```python
from build123d import *

# Parameters (mm, degrees)
BOSS_EXTRUDE1_DEPTH = 300
BOSS_EXTRUDE2_DEPTH = 10
SKETCH3_R           = 5
CUT_EXTRUDE1_DEPTH  = 624.643527987


with BuildPart() as part:
    # Sketch1 → Boss-Extrude1 (new, symmetric)
    with BuildSketch(Plane(origin=(0, 0, 0), x_dir=(0, 0, -1), z_dir=(1, 0, 0))):
        with BuildLine():
            Line((-20, 25), (20, 25))
            ThreePointArc((20, 25), (23.535533906, 23.535533906), (25, 20))
            Line((25, 20), (25, -20))
            ThreePointArc((25, -20), (23.535533906, -23.535533906), (20, -25))
            Line((20, -25), (-20, -25))
            ThreePointArc((-20, -25), (-23.535533906, -23.535533906), (-25, -20))
            Line((-25, -20), (-25, 20))
            ThreePointArc((-25, 20), (-23.535533906, 23.535533906), (-20, 25))
        make_face()
        with BuildLine():
            Line((-20, 23), (20, 23))
            ThreePointArc((20, 23), (22.121320344, 22.121320344), (23, 20))
            Line((23, 20), (23, -20))
            ThreePointArc((23, -20), (22.121320344, -22.121320344), (20, -23))
            Line((20, -23), (-20, -23))
            ThreePointArc((-20, -23), (-22.121320344, -22.121320344), (-23, -20))
            Line((-23, -20), (-23, 20))
            ThreePointArc((-23, 20), (-22.121320344, 22.121320344), (-20, 23))
        make_face(mode=Mode.SUBTRACT)
    extrude(amount=BOSS_EXTRUDE1_DEPTH, both=True)

    # Sketch2 → Boss-Extrude2 (add)
    with BuildSketch(Plane(origin=(300, 0, 0), x_dir=(0, 0, -1), z_dir=(1, 0, 0))):
        with BuildLine():
            Line((-57.5, 25), (57.5, 25))
            ThreePointArc((57.5, 25), (61.035533906, 23.535533906), (62.5, 20))
            Line((62.5, 20), (62.5, -20))
            ThreePointArc((62.5, -20), (61.035533906, -23.535533906), (57.5, -25))
            Line((57.5, -25), (-57.5, -25))
            ThreePointArc((-57.5, -25), (-61.035533906, -23.535533906), (-62.5, -20))
            Line((-62.5, -20), (-62.5, 20))
            ThreePointArc((-62.5, 20), (-61.035533906, 23.535533906), (-57.5, 25))
        make_face()
    boss_extrude2 = extrude(amount=BOSS_EXTRUDE2_DEPTH)

    # Mirror1: Boss-Extrude2 across plane
    add(boss_extrude2.mirror(Plane(origin=(0, 0, 0), x_dir=(0, 0, 1), z_dir=(1, 0, 0))))

    # Sketch3 → Cut-Extrude1 (cut, through all)
    with BuildSketch(Plane(origin=(310, 0, 0), x_dir=(0, 0, -1), z_dir=(1, 0, 0))):
        with Locations((-47.5, 0)):
            Circle(SKETCH3_R)
        with Locations((47.5, 0)):
            Circle(SKETCH3_R)
    extrude(amount=-CUT_EXTRUDE1_DEPTH, mode=Mode.SUBTRACT)


solid = part.part
```
The listing builds one solid part. Answer for the finished solid, in the listing's coordinates (mm). A direction names the side the tool comes from. Give positions to 0.01 mm unless a question says otherwise; leave off trailing zeros. Order: outer loops, then holes, each group sorted by start corner. A loop starts at its lowest first (then second) coordinate and runs counter-clockwise, first axis right, second up. Notation, with made-up numbers: (0.5, 44) - (49.5, 44) arc R24 cw to (49.5, 79) - close; hole circle Ø5 at (8, -8.75). An arc over 180 degrees is marked (long way). Answer in a Markdown table with one row per item. Add a question column.
Q1. Find the intervals of material crossed by line 1 along X through (y, z) = (7.5, 15.5); line 2 along Z through (x, y) = (-34, 17.5), in increasing order. Write a range as [from, to].
Q2. The part is cut by section B-B (x = -14). Determine the outline of the cut face in (y, z).
Q3. The part is cut by section A-A (z = 14). Determine the outline of the cut face in (x, y), then the cut area to 3 significant figures.
Q4. For a pull along X with two mould halves and no side action, classify faces 1 (the flat face through (1, 25, 9)), 2 (the flat face through (-300, 0, 41)), 3 (the flat face through (310, 0, -1)) as released by +X, released by -X, zero draft, split by the parting line, or undercut.
Q5. Given P1, Ø12, axis at x = 145.5, y = 8.5, coming from the +Z side; P2, Ø6, axis at x = -148.5, y = 0.5, coming from the -Z side; P3, Ø6, axis at y = 0, z = -47.5, coming from the -X side, each flat-ended and moving along its own axis, determine where each tip first touches the part or whether it passes through.
Q6. Which of the six approach directions +Z, -Z, +X, -X, +Y, -Y give full straight-line access (tool end or side, diameter ignored) to faces 4 (the flat face through (-305, 0, -62.5)), 5 (the flat face through (4, 0, -25)), 6 (the cylindrical face through (-304.93, 0.22, -42.505)), 7 (the flat face through (4, 0, 25)), 8 (the flat face through (4, 23, 0))?
Determined:
| question | item | result |
|---|---|---|
| 1 | line 1 | x = [-310, -300], [300, 310] |
| 1 | line 2 | z = [-25, -23], [23, 25] |
| 2 | outline | (-25, -20) arc R5 ccw to (-20, -25) - (20, -25) arc R5 ccw to (25, -20) - (25, 20) arc R5 ccw to (20, 25) - (-20, 25) arc R5 ccw to (-25, 20) - close; hole (-23, -20) arc R3 ccw to (-20, -23) - (20, -23) arc R3 ccw to (23, -20) - (23, 20) arc R3 ccw to (20, 23) - (-20, 23) arc R3 ccw to (-23, 20) - close |
| 3 | outline | (-310, -25) - (310, -25) - (310, 25) - (-310, 25) - close; hole (-300, -23) - (300, -23) - (300, 23) - (-300, 23) - close |
| 3 | area | 3,400 mm² |
| 4 | face 1 | zero draft |
| 4 | face 2 | undercut |
| 4 | face 3 | released by +X |
| 5 | P1 | stops at z = 25 |
| 5 | P2 | stops at z = -25 |
| 5 | P3 | passes through |
| 6 | face 4 | -Z, +X, -X, +Y, -Y |
| 6 | face 5 | -Z, +Y, -Y |
| 6 | face 6 | +X, -X |
| 6 | face 7 | +Z, +Y, -Y |
| 6 | face 8 | none |
